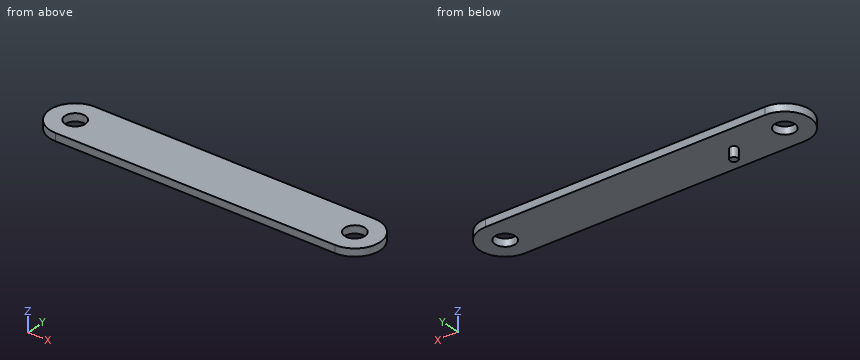
from build123d import *

# Parameters (mm, degrees)
SKETCH1_R           = 4.01
BOSS_EXTRUDE1_DEPTH = 3
SKETCH2_R           = 1.49
BOSS_EXTRUDE3_DEPTH = 4


with BuildPart() as part:
    # Sketch1 → Boss-Extrude1 (new body)
    with BuildSketch(Plane.XY):
        with BuildLine():
            Line((110, 10), (0, 10))
            ThreePointArc((0, 10), (-10, 0), (0, -10))
            Line((0, -10), (110, -10))
            ThreePointArc((110, -10), (120, 0), (110, 10))
        make_face()
        Circle(SKETCH1_R, mode=Mode.SUBTRACT)
        with Locations((110, 0)):
            Circle(SKETCH1_R, mode=Mode.SUBTRACT)
    extrude(amount=BOSS_EXTRUDE1_DEPTH)

    # Sketch2 → Boss-Extrude3 (add)
    with BuildSketch(Plane(origin=(0, 0, 0), x_dir=(-1, 0, 0), z_dir=(0, 0, -1))):
        with Locations(Location((-20, 0, 0), (0, 0, 180))):
            Circle(SKETCH2_R)
    extrude(amount=BOSS_EXTRUDE3_DEPTH)


solid = part.part
Can you work these out from the model? Positions are in its coordinate system, mm. Coordinates: 2 decimals unless noted, no trailing zeros. Order: outer loops, then holes, each group sorted by start corner. A loop starts at its lowest first (then second) coordinate and runs counter-clockwise, first axis right, second up. Notation, with made-up numbers: M -40,31 L 5,31 A22 cw 5,70 Z; hole C 52.25,1.5 d4. An arc over 180 degrees is marked long. Write item = value, one per line.
(1) Suppose I cut it at C-C on z = -2.5. Please give me the cut outline in (x, y).
Results are:
outline = C 20,0 d2.98
(2) Suppose I cut it at A-A on y = 0. Please give me the cut outline in (x, z), plus the area to 3 significant figures.
Results are:
outline = M -10,0 L -4.01,0 L -4.01,3 L -10,3 Z; M 4.01,0 L 18.51,0 L 18.51,-4 L 21.49,-4 L 21.49,0 L 105.99,0 L 105.99,3 L 4.01,3 Z; M 114.01,0 L 120,0 L 120,3 L 114.01,3 Z
area = 354 mm2
(3) For pin 1 Ø6 at (x, y) = (30.5, -4.5) entering from -Z; pin 2 Ø2 at (x, z) = (6.5, -0.5) entering from +Y; pin 3 Ø4 at (y, z) = (5.5, -1) entering from -X; pin 4 Ø3 at (y, z) = (-6.5, 2) entering from +X, each with a flat end and sliding along its axis, tell me the tip position at first contact or that it passes through.
Results are:
pin_1 = 0
pin_2 = 10
pin_3 = -9.26
pin_4 = 118.66
(4) Suppose I cut it at D-D on y = -6.25. Please give me the cut outline in (x, z), plus the area to 3 significant figures.
Results are:
outline = M -7.81,0 L 117.81,0 L 117.81,3 L -7.81,3 Z
area = 377 mm2
(5) Suppose I cut it at B-B on x = 20. Please give me the cut outline in (y, z), plus the area to 3 significant figures.
Results are:
outline = M -10,0 L -1.49,0 L -1.49,-4 L 1.49,-4 L 1.49,0 L 10,0 L 10,3 L -10,3 Z
area = 71.9 mm2
(6) I need wall thicknesses on line 1 along X through (y, z) = (-0.25, 1.25); line 2 along Y through (x, z) = (0, 2.3); line 3 along X through (y, z) = (1.25, 2). Which ranges of each line are inside material? Lowest first, please. Write a range as [from, to].
Results are:
line_1 = [-10, -4], [4, 106], [114, 120]
line_2 = [-10, -4.01], [4.01, 10]
line_3 = [-9.92, -3.81], [3.81, 106.19], [113.81, 119.92]
